from build123d import *

# Parameters (mm, degrees)
CROQUIS1_R              = 4.1
CROQUIS1_R_2            = 4
SALIENTE_EXTRUIR1_DEPTH = 4
CROQUIS2_R              = 10.5
CORTAR_EXTRUIR1_DEPTH   = 1.5
CROQUIS3_R              = 0.75
CORTAR_EXTRUIR2_DEPTH   = 10


with BuildPart() as part:
    # Croquis1 → Saliente-Extruir1 (new body)
    with BuildSketch(Plane(origin=(0, 0, 0), x_dir=(0, 0, -1), z_dir=(1, 0, 0))):
        with BuildLine():
            Line((-70.267857143, 12.497129773), (-0.3, 13.996785345))
            ThreePointArc((-0.3, 13.996785345), (14, 0), (-0.3, -13.996785345))
            Line((-0.3, -13.996785345), (-70.267857143, -12.497129773))
            ThreePointArc((-70.267857143, -12.497129773), (-82.5, 0), (-70.267857143, 12.497129773))
        make_face()
        Circle(CROQUIS1_R, mode=Mode.SUBTRACT)
        with Locations((-70, 0)):
            Circle(CROQUIS1_R_2, mode=Mode.SUBTRACT)
    extrude(amount=SALIENTE_EXTRUIR1_DEPTH)

    # Croquis2 → Cortar-Extruir1 (cut)
    with BuildSketch(Plane(origin=(4, 0, 0), x_dir=(0, 0, -1), z_dir=(1, 0, 0))):
        with Locations((-70, 0)):
            Circle(CROQUIS2_R)
    extrude(amount=-CORTAR_EXTRUIR1_DEPTH, mode=Mode.SUBTRACT)

    # Croquis3 → Cortar-Extruir2 (cut)
    with BuildSketch(Plane.ZY):
        with Locations((63.65189161, -5.658093307)):
            Circle(CROQUIS3_R)
        with Locations((76.34810839, 5.658093307)):
            Circle(CROQUIS3_R)
        with Locations((64.341906693, 6.34810839)):
            Circle(CROQUIS3_R)
        with Locations((75.658093307, -6.34810839)):
            Circle(CROQUIS3_R)
    extrude(amount=-CORTAR_EXTRUIR2_DEPTH, mode=Mode.SUBTRACT)


solid = part.part
Geometry check sheet. Reference: the model listing, model coordinates, mm. Coordinates: 2 decimals unless noted, no trailing zeros. Order: outer loops, then holes, each group sorted by start corner. A loop starts at its lowest first (then second) coordinate and runs counter-clockwise, first axis right, second up. Notation, with made-up numbers: (-28, 54.25) - (21, 54.25) arc R26 ccw to (21, 84.25) - close; hole circle Ø7 at (27, -30.5). An arc over 180 degrees is marked (long way). Answer in a Markdown table with one row per item. Add a question column.
1) Material ranges on line 1 along Y through (x, z) = (2, 0); line 2 along Y through (x, z) = (1.7, 70); line 3 along Z through (x, y) = (2.2, -0.75), recorded low to high. Write a range as [from, to].
2) Cross-section at B-B, the plane x = 1.3. Record the cut outline in (y, z).
3) Release check for a two-part mould opening along Y. For faces 1 (the flat face through (0, 0, 34)), 2 (the cylindrical face through (1.972, -0.271, 82.497)), 3 (the cylindrical face through (3.26, 7.096, 77.739)), 4 (the flat face through (2.5, 0, 65)) record: +Y half, -Y half, draft (parallel to the pull), parting line (faces both ways), or undercut.
4) Cross-section at A-A, the plane y = 0. Record the cut outline in (x, z).
5) Gauge pin test, flat ends, axial feed: P1, Ø2, axis at y = 6.35, z = 64.34, coming from the -X side; P2, Ø1.2, axis at y = -5.66, z = 63.65, coming from the +X side; P3, Ø2.5, axis at y = -6.35, z = 75.66, coming from the +X side. Record the tip position at first contact, or that the pin passes through.
6) Cross-section at C-C, the plane y = -8.75. Record the cut outline in (x, z).
7) Cross-section at D-D, the plane z = 24.5. Record the cut outline in (x, y), then the cut area to 3 significant figures.
Check result:
| question | item | result |
|---|---|---|
| 1 | line 1 | y = [-14, -4.1], [4.1, 14] |
| 1 | line 2 | y = [-12.5, -4], [4, 12.5] |
| 1 | line 3 | z = [-13.98, -4.03], [4.03, 66.07], [73.93, 82.48] |
| 2 | outline | (-14, 0.3) arc R14 ccw (long way) to (14, 0.3) - (12.5, 70.27) arc R12.5 ccw to (-12.5, 70.27) - close; hole circle Ø1.5 at (-6.35, 75.66); hole circle Ø1.5 at (-5.66, 63.65); hole circle Ø8.2 at (0, 0); hole circle Ø8 at (0, 70); hole circle Ø1.5 at (5.66, 76.35); hole circle Ø1.5 at (6.35, 64.34) |
| 3 | face 1 | draft |
| 3 | face 2 | parting line |
| 3 | face 3 | undercut |
| 3 | face 4 | undercut |
| 4 | outline | (0, -14) - (4, -14) - (4, -4.1) - (0, -4.1) - close; (0, 4.1) - (4, 4.1) - (4, 59.5) - (2.5, 59.5) - (2.5, 66) - (0, 66) - close; (0, 74) - (2.5, 74) - (2.5, 80.5) - (4, 80.5) - (4, 82.5) - (0, 82.5) - close |
| 5 | P1 | stops at x = 0 |
| 5 | P2 | passes through |
| 5 | P3 | stops at x = 2.5 |
| 6 | outline | (0, -10.93) - (4, -10.93) - (4, 64.2) - (2.5, 64.2) - (2.5, 75.8) - (4, 75.8) - (4, 78.93) - (0, 78.93) - close |
| 7 | outline | (0, -13.48) - (4, -13.48) - (4, 13.48) - (0, 13.48) - close |
| 7 | area | 108 mm² |
